Geometry: see drawing. Coordinates: mm, zero at the bounding-box minimum. Give positions to 0.01 mm unless a question says otherwise; leave off trailing zeros. Write item = value, one per line.
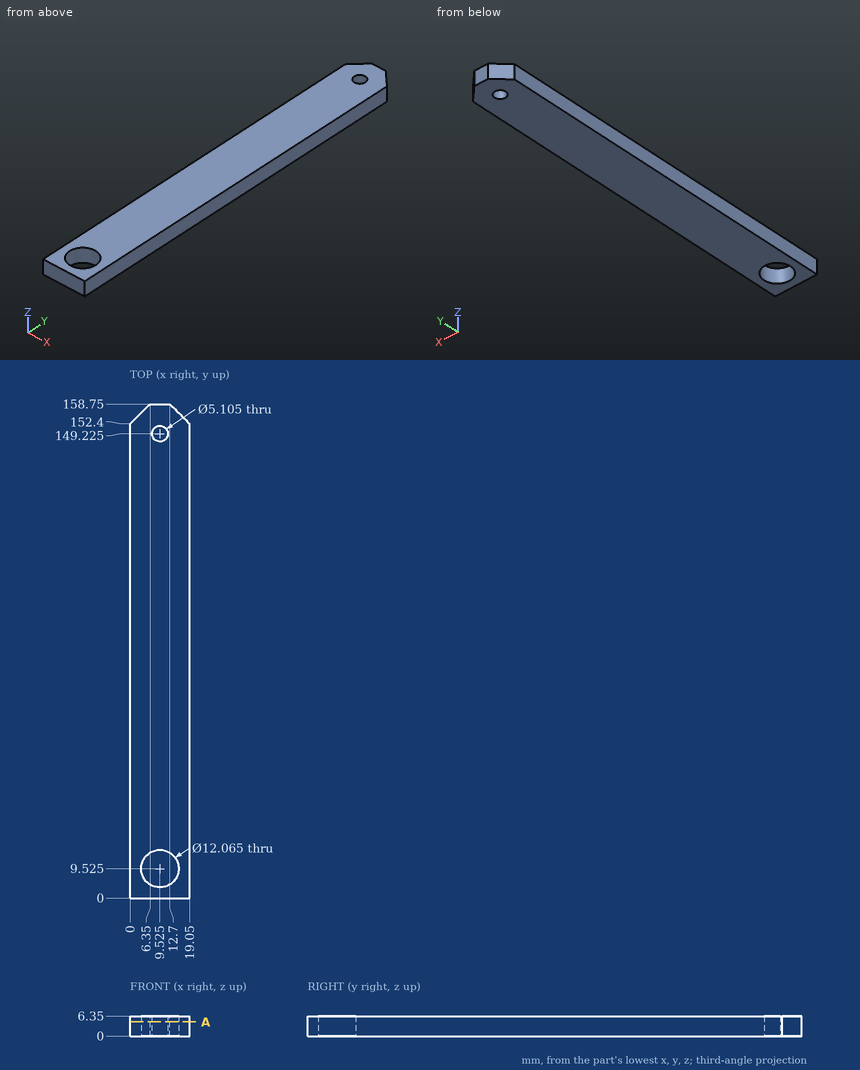
(1) Material intervals for line 1 (X direction, y = 10, z = 5.75); line 2 (Y direction, x = 8.5, z = 2.5); line 3 (Y direction, x = 10, z = 4.5), sorted ascending.
Values follow:
line_1 = 0 to 3.51, 15.54 to 19.05
line_2 = 0 to 3.58, 15.47 to 146.89, 151.56 to 158.75
line_3 = 0 to 3.51, 15.54 to 146.72, 151.73 to 158.75
(2) First-contact query: pin 1 (9.5 mm diameter, centred on x = 9.525, y = 9.525, fed in from +Z); pin 2 (3 mm diameter, centred on x = 14.5, y = 48.5, fed in from -Z). Flat tips, straight axial feed; report the tip coordinate or a pass-through.
Values follow:
pin_1 = through
pin_2 = 0
(3) Section query A-A (z = 4.5). Give the number of separate pieces and of enclosed holes in the cut face, plus the area to 3 significant figures.
Values follow:
separate_pieces = 1
enclosed_holes = 2
area = 2,850 mm2
